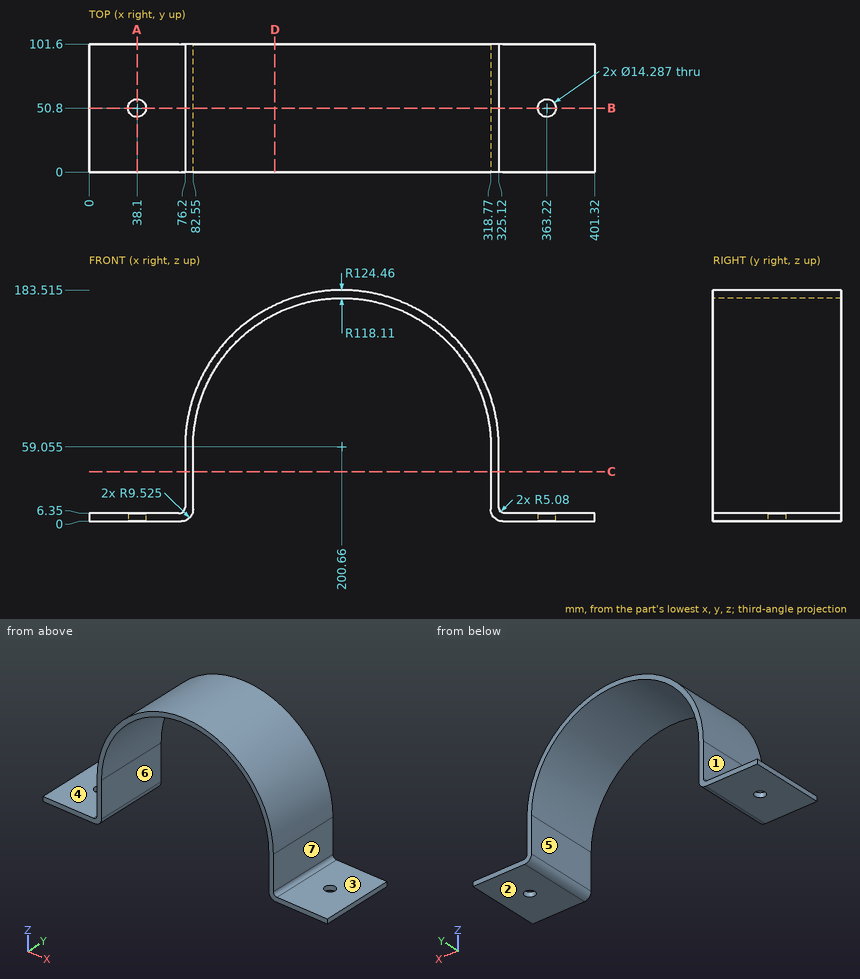
Can you work these out from the drawing? Everything is in mm from the part's minimum corner. A direction names the side the tool comes from. Coordinates: 2 decimals unless noted, no trailing zeros. Write each loop counter-clockwise with the first axis right and the second up, starting at its lowest first coordinate (ties: lowest second). Pieces come first, ordered by that corner, then holes. Notation, with made-up numbers: (62.5, -22.75) -> (92.5, -22.75) arc R17 cw to (92.5, -4.75) -> close; hole circle Ø4 at (20, 66). An arc over 180 degrees is marked (long way). Return JSON: item names as keys, results as strings.
(1) Which directions (+Z, -Z, +X, -X, +Y, -Y) give clear straight access to the entire face, cutting with the end or side of a thin tool? Please do the marked faces 1, 2 and 3.
Numbers:
{"face 1": "+Z, -X, +Y, -Y", "face 2": "-Z, +X, -X, +Y, -Y", "face 3": "+Z, +X, +Y, -Y"}
(2) Imagine slicing it at D-D, the plane x = 147.5. Please give me the cut outline in (y, z) (1 decimal).
Numbers:
{"outline": "(0, 164.5) -> (101.6, 164.5) -> (101.6, 171.6) -> (0, 171.6) -> close"}
(3) Imagine slicing it at C-C, the plane z = 39.5. Please give me the cut outline in (x, y).
Numbers:
{"outline": "(76.2, 0) -> (82.55, 0) -> (82.55, 101.6) -> (76.2, 101.6) -> close; (318.77, 0) -> (325.12, 0) -> (325.12, 101.6) -> (318.77, 101.6) -> close"}
(4) Imagine slicing it at B-B, the plane y = 50.8. Count the separate pieces of the cut face and the enclosed holes in it, then the cut area to 3 significant figures.
Numbers:
{"separate pieces": "3", "enclosed holes": "0", "area": "3,930 mm2"}
(5) I'm going to push flat-ended pins straight in: pin 1 (14.5 mm diameter, centred on y = 71, z = 35.5, fed in from -X); pin 2 (8.5 mm diameter, centred on x = 38.1, y = 50.8, fed in from -Z); pin 3 (6 mm diameter, centred on x = 158.5, y = 77.5, fed in from +Z); pin 4 (14.5 mm diameter, centred on y = 67.5, z = 26, fed in from +X). Where does each tip first touch, or does it pass through?
Numbers:
{"pin 1": "stops at x = 76.2", "pin 2": "passes through", "pin 3": "stops at z = 177.19", "pin 4": "stops at x = 325.12"}
(6) Imagine slicing it at A-A, the plane x = 38.1. Please give me the cut outline in (y, z).
Numbers:
{"outline": "(0, 0) -> (43.66, 0) -> (43.66, 6.35) -> (0, 6.35) -> close; (57.94, 0) -> (101.6, 0) -> (101.6, 6.35) -> (57.94, 6.35) -> close"}
(7) I need wall thicknesses on L1, parallel to X at y = 75, z = 46.5; L2, parallel to X at y = 50.8, z = 2 (1 decimal); L3, parallel to Y at x = 363.22, z = 1.5. Which ranges of each line are inside material? Lowest first, please.
Numbers:
{"L1": "x = 76.2 to 82.55, 318.77 to 325.12", "L2": "x = 0 to 31, 45.2 to 78.9, 322.5 to 356.1, 370.4 to 401.3", "L3": "y = 0 to 43.66, 57.94 to 101.6"}
(8) We'd pull the mould along X, two halves only. Please class the marked faces 4, 5, 6 and 7: +X half, -X half, draft (parallel to the pull), parting line (faces both ways), or undercut.
Numbers:
{"face 4": "draft", "face 5": "undercut", "face 6": "undercut", "face 7": "+X half"}
